```python
from build123d import *

# Parameters (mm, degrees)
SKETCH1_R               = 3
BOSS_EXTRUDE1_DEPTH     = 3.5
SKETCH2_R               = 4
BOSS_EXTRUDE2_DEPTH     = 2
SKETCH3_R               = 2
CUT_EXTRUDE1_DEPTH      = 8
SKETCH4_R               = 1
CUT_EXTRUDE2_DEPTH      = 5
CUT_EXTRUDE2_DEPTH_BACK = 5


with BuildPart() as part:
    # Sketch1 → Boss-Extrude1 (new body, symmetric)
    with BuildSketch(Plane(origin=(0, 0, 0), x_dir=(0, 0, -1), z_dir=(1, 0, 0))):
        Circle(SKETCH1_R)
    extrude(amount=BOSS_EXTRUDE1_DEPTH, both=True)

    # Sketch2 → Boss-Extrude2 (add)
    with BuildSketch(Plane.ZY.offset(3.5)):
        Circle(SKETCH2_R)
    extrude(amount=-BOSS_EXTRUDE2_DEPTH)

    # Sketch3 → Cut-Extrude1 (cut, through all)
    with BuildSketch(Plane(origin=(3.5, 0, 0), x_dir=(0, 0, -1), z_dir=(1, 0, 0))):
        Circle(SKETCH3_R)
    extrude(amount=-CUT_EXTRUDE1_DEPTH, mode=Mode.SUBTRACT)

    # Sketch4 → Cut-Extrude2 (cut, two sides)
    with BuildSketch(Plane(origin=(0, 0, 0), x_dir=(1, 0, 0), z_dir=(0, 1, 0))) as cut_extrude2_sk:
        with Locations((1, 0)):
            Circle(SKETCH4_R)
    extrude(amount=CUT_EXTRUDE2_DEPTH, mode=Mode.SUBTRACT)
    extrude(cut_extrude2_sk.sketch, amount=-CUT_EXTRUDE2_DEPTH_BACK, mode=Mode.SUBTRACT)


solid = part.part
```
Geometry check sheet. Reference: the model listing, model coordinates, mm. A direction names the side the tool comes from. Round coordinates to 2 decimals unless told otherwise and drop trailing zeros. Order: outer loops, then holes, each group sorted by start corner. A loop starts at its lowest first (then second) coordinate and runs counter-clockwise, first axis right, second up. Notation, with made-up numbers: (49.25, 83.25) - (63.25, 83.25) arc R16 ccw to (63.25, 105.25) - close; hole circle Ø1 at (88.25, -12.5). An arc over 180 degrees is marked (long way). Use a Markdown table: item, result. Add a question column.
(1) Sectioned sample at D-D, the plane x = 0.5. Enter the section's corners in (y, z).
(2) Sectioned sample at A-A, the plane z = 0. Enter the section's corners in (x, y).
(3) Sectioned sample at C-C, the plane x = -0.5. Enter the section's corners in (y, z), and give its area (3 significant figures).
(4) Material ranges on line 1 along Y through (x, z) = (-0.5, 0); line 2 along Z through (x, y) = (1, -2.45); line 3 along X through (y, z) = (2.15, 0), recorded low to high. Write a range as [from, to].
(5) Depth check by flat-ended pin: pin 1 (1 mm diameter, centred on x = -2, z = 3, fed in from -Y); pin 2 (1.6 mm diameter, centred on x = 1, z = 0, fed in from +Y); pin 3 (3 mm diameter, centred on x = 1, z = 0, fed in from +Y); pin 4 (1 mm diameter, centred on x = 1, z = 2, fed in from -Y). Enter the tip coordinate at first touch or a pass-through.
(6) Tool access check on faces 4 (the flat face through (3.5, -2, -1)), 5 (the flat face through (-1.5, 3, 1)). Record the directions out of +Z, -Z, +X, -X, +Y, -Y that give a thin tool (end or side, any length) a straight path to the whole face; none if there is none.
(7) Release check for a two-part mould opening along Z. For faces 1 (the cylindrical face through (-2.514, -3.905, -0.867)), 2 (the flat face through (-3.5, -1, -2)), 3 (the cylindrical face through (0.2, 2.4, 0.6)) record: pulls with the +Z half, pulls with the -Z half, needs draft (parallel to the pull), parting line crosses it, or undercut.
(8) Sectioned sample at B-B, the plane y = 0. Enter the section's corners in (x, z).
Answers below:
| question | item | result |
|---|---|---|
| 1 | outline | (-2.87, -0.87) arc R3 ccw to (2.87, -0.87) - (1.8, -0.87) arc R2 cw to (-1.8, -0.87) - close; (-2.87, 0.87) - (-1.8, 0.87) arc R2 cw to (1.8, 0.87) - (2.87, 0.87) arc R3 ccw to start |
| 2 | outline | (-3.5, -4) - (-1.5, -4) - (-1.5, -3) - (0, -3) - (0, -2) - (-3.5, -2) - close; (-3.5, 2) - (0, 2) - (0, 3) - (-1.5, 3) - (-1.5, 4) - (-3.5, 4) - close; (2, -3) - (3.5, -3) - (3.5, -2) - (2, -2) - close; (2, 2) - (3.5, 2) - (3.5, 3) - (2, 3) - close |
| 3 | outline | circle Ø6 at (0, 0); hole circle Ø4 at (0, 0) |
| 3 | area | 15.7 mm² |
| 4 | line 1 | [-3, -2], [2, 3] |
| 4 | line 2 | [-1.73, -1], [1, 1.73] |
| 4 | line 3 | [-3.5, 0], [2, 3.5] |
| 5 | pin 1 | y = -3.12 |
| 5 | pin 2 | through |
| 5 | pin 3 | y = 3 |
| 5 | pin 4 | y = -2.6 |
| 6 | face 4 | +Z, -Z, +X, +Y, -Y |
| 6 | face 5 | +X |
| 7 | face 1 | parting line crosses it |
| 7 | face 2 | needs draft |
| 7 | face 3 | undercut |
| 8 | outline | (-3.5, -4) - (-1.5, -4) - (-1.5, -3) - (3.5, -3) - (3.5, -2) - (-3.5, -2) - close; (-3.5, 2) - (3.5, 2) - (3.5, 3) - (-1.5, 3) - (-1.5, 4) - (-3.5, 4) - close |
